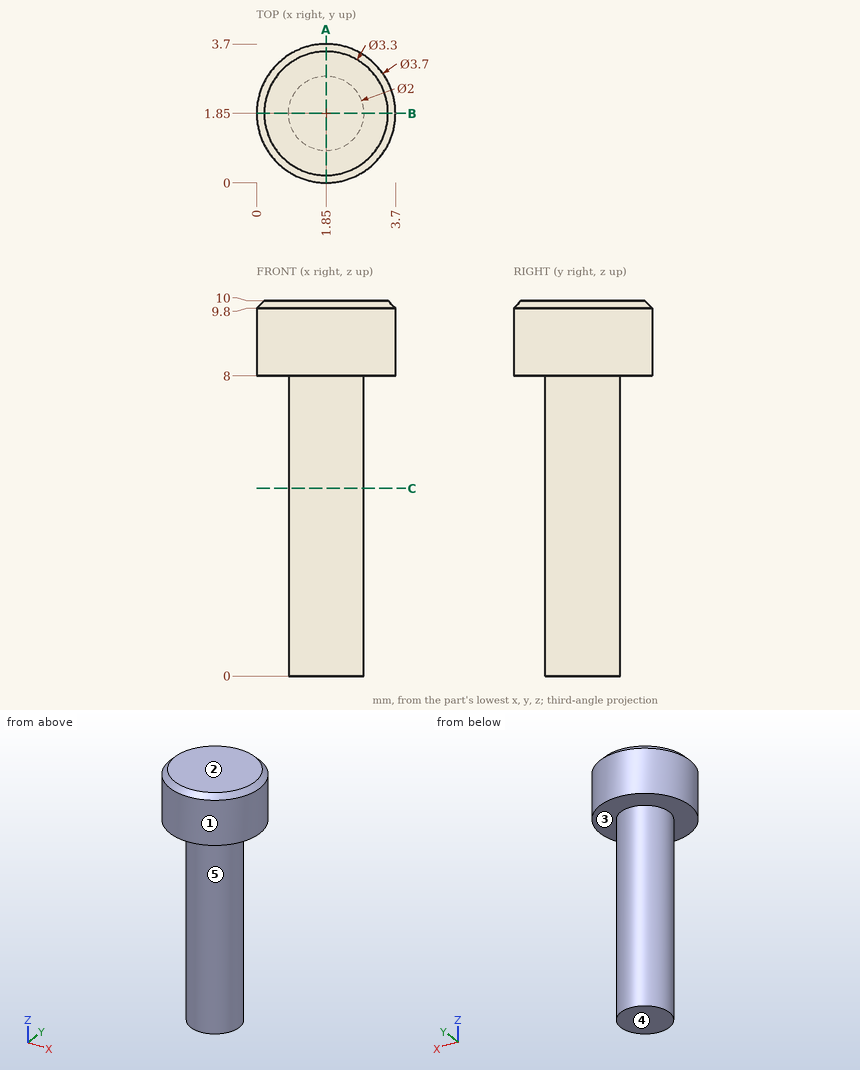
The drawing under review shows one solid part. Ordinate dimensions are in mm from its lowest x, y, z. A direction names the side the tool comes from. Give positions to 0.01 mm unless a question says otherwise; leave off trailing zeros. Order: outer loops, then holes, each group sorted by start corner. A loop starts at its lowest first (then second) coordinate and runs counter-clockwise, first axis right, second up. Notation, with made-up numbers: (63.25, 35.5) - (103.25, 35.5) arc R10 ccw to (103.25, 51.5) - close; hole circle Ø9 at (-3, 81.5). An arc over 180 degrees is marked (long way). Answer as a JSON object with one key per item and string values. Group by question number.
Item 1: Clearance check with a flat-ended pin moving along its axis: pin 1 Ø1 at (x, z) = (2.5, 5.5) entering from -Y. State where the tip first meets the part, or that it passes through.
Item 2: Wall thickness on line 1 along Z through (x, y) = (2.15, 3.3); line 2 along X through (y, z) = (1.8, 1.5): over which ranges is each line inside the solid? List them lowest first.
Item 3: Take a section at A-A on x = 1.85. Give the boundary of the cut face in (y, z), and give its area (3 significant figures).
Item 4: Take a section at C-C on z = 5. Give the boundary of the cut face in (x, y), and give its area (3 significant figures).
Item 5: Draft analysis for pull direction Z (two halves, no side actions). For the marked faces 1, 2 and 3, state which applies: pulls with the +Z half, pulls with the -Z half, needs draft (parallel to the pull), parting line crosses it, or undercut.
Item 6: Machinability: for the marked faces 4 and 5, which of the approach directions +Z, -Z, +X, -X, +Y, -Y give a long, thin tool a straight path to every point of the face, cutting with its end or side? Answer none if there is none.
Reported:
{
 "1": {"pin 1": "y = 0.86"},
 "2": {"line 1": "8 to 10", "line 2": "0.85 to 2.85"},
 "3": {"outline": "(0, 8) - (0.85, 8) - (0.85, 0) - (2.85, 0) - (2.85, 8) - (3.7, 8) - (3.7, 9.8) - (3.5, 10) - (0.2, 10) - (0, 9.8) - close", "area": "23.4 mm^2"},
 "4": {"outline": "circle Ø2 at (1.85, 1.85)", "area": "3.14 mm^2"},
 "5": {"face 1": "needs draft", "face 2": "pulls with the +Z half", "face 3": "pulls with the -Z half"},
 "6": {"face 4": "-Z, +X, -X, +Y, -Y", "face 5": "-Z"}
}
